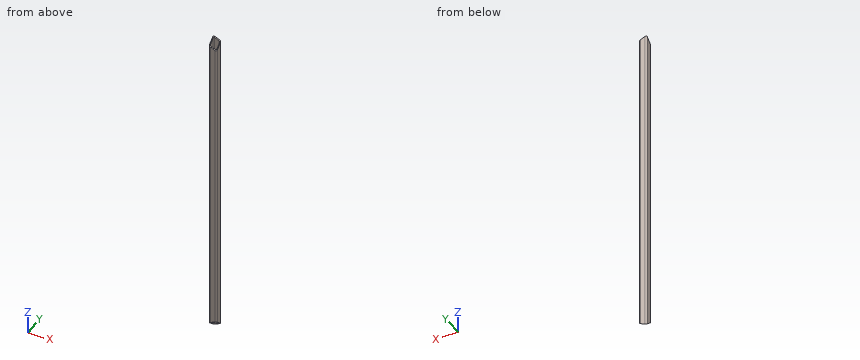
Autodesk Inventor part; units mm, degrees
ref_plane "Plano inicial" through (0, 0, -34.0777) normal (0, 0, 1) x (1, 0, 0)
ref_plane "Plano final" through (0, 0, 2032.731) normal (0, 0, 1) x (1, 0, 0)
ref_plane "Plano de trabalho4" through (-13.7846, 27.5692, -30.8233) normal (0.3162, -0.6325, -0.7071) x (0.6586, 0.6828, -0.3162)
ref_plane "Plano inicial" through (0, 0, -34.0777) normal (0, 0, 1) x (1, 0, 0)
ref_plane "Plano final" through (0, 0, 2032.731) normal (0, 0, 1) x (1, 0, 0)
sketch "Esboço" plane through (0, 0, 0) normal (0, 0, 1) x (1, 0, 0)
  line L0 (-25.4, -15.875) -> (-25.4, 15.875)
  line L1 (-15.875, 25.4) -> (15.875, 25.4)
  line L2 (25.4, 15.875) -> (25.4, -15.875)
  line L3 (15.875, -25.4) -> (-15.875, -25.4)
  arc A0 (-25.4, -15.875) -> (-15.875, -25.4) centre (-15.875, -15.875) ccw
  arc A1 (-15.875, 25.4) -> (-25.4, 15.875) centre (-15.875, 15.875) ccw
  arc A2 (25.4, 15.875) -> (15.875, 25.4) centre (15.875, 15.875) ccw
  arc A3 (15.875, -25.4) -> (25.4, -15.875) centre (15.875, -15.875) ccw
  arc A4 (-15.875, 20.6375) -> (-20.6375, 15.875) centre (-15.875, 15.875) ccw
  line L4 (-15.875, 20.6375) -> (15.875, 20.6375)
  arc A5 (20.6375, 15.875) -> (15.875, 20.6375) centre (15.875, 15.875) ccw
  line L5 (20.6375, 15.875) -> (20.6375, -15.875)
  arc A6 (15.875, -20.6375) -> (20.6375, -15.875) centre (15.875, -15.875) ccw
  line L6 (15.875, -20.6375) -> (-15.875, -20.6375)
  arc A7 (-20.6375, -15.875) -> (-15.875, -20.6375) centre (-15.875, -15.875) ccw
  line L7 (-20.6375, -15.875) -> (-20.6375, 15.875)
  line L8 (0, 38.3218) -> (0, -38.3218) construction
  line L9 (-38.3218, 0) -> (38.3218, 0) construction
  dimension "d10" = 50.8
  dimension "d11" = 50.8
  dimension "d12" = 4.7625
  dimension "d15" = 25.4
  dimension "d16" = 25.4
  dimension "d17" = 9.525
extrude "Corpo" add sketch "Esboço" along normal up to surface (2066.8087 mm away) from surface at -34.0777
sketch "Sketch3" plane through (0, 0, 0) normal (0, 0, 1) x (1, 0, 0)
  line L0 (0, 0) -> (10, 0)
ref_plane "Work Plane3" through (0, 0, 0) normal (0, -1, 0) x (1, 0, 0)
sketch "Sketch4" plane through (0, 0, 0) normal (0, -1, 0) x (1, 0, 0)
  line L0 (-2, -34.0777) -> (12, -34.0777)
  line L1 (-2, 2032.731) -> (12, 2032.731)
  dimension "d19" = 2066.8087
ref_plane "Plano de trabalho4" through (-13.7846, 27.5692, -30.8233) normal (0.3162, -0.6325, -0.7071) x (0.6586, 0.6828, -0.3162)
split "Dividir1" plane through (-13.7846, 27.5692, -30.8233) removes the side toward (0.3162, -0.6325, -0.7071)
ref_plane "Plano de trabalho5" through (-13.7846, 27.5692, 2029.6052) normal (0.3098, -0.6196, 0.7212) x (0.9442, 0.1115, -0.3098)
split "Dividir2" plane through (-13.7846, 27.5692, 2029.6052) removes the side toward (0.3098, -0.6196, 0.7212)
equation "\"d10\" = G_H"
equation "\"d11\" = G_W"
equation "\"d12\" = G_T"
equation "\"d15\" = 0.5 * d10"
equation "\"d16\" = 0.5 * d11"
equation "\"d17\" = G_IR"
equation "\"d3\" = G_L"
equation "\"G_W\" = 50.8"
equation "\"G_H\" = 50.8"
equation "\"G_T\" = 4.7625"
equation "\"G_IR\" = 9.525"
equation "\"G_L\" = 2060.38202"
equation "\"G_OFFSET_START\" = 34.07768"
equation "\"G_OFFSET_END\" = 32.73098"
equation "\"d13\" = -G_OFFSET_START"
equation "\"d14\" = G_OFFSET_END + B_L"
properties part number "AISC - 2 x 2 x 3/16 - 81,117" material "Aço, suave"
CAD build for the part. Positions are in the model's coordinates, mm. Coordinates: 2 decimals unless noted, no trailing zeros. Loops run counter-clockwise (first coordinate to the right, second up) from the corner with the lowest first, then second, coordinate; pieces in that order, holes last. Notation, with made-up numbers: (31.5, 33.25) -> (67.5, 33.25) arc R9 cw to (67.5, 47.25) -> close; hole circle Ø11 at (61.25, 74.5). An arc over 180 degrees is marked (long way). One line per item, written item: value.
1. Drill centre lines: line 1 (X direction, y = 16.5, z = 259); line 2 (Y direction, x = -14, z = 1445); line 3 (X direction, y = 22, z = 1805.5). Where is each one in solid material? Low to high. Write a range as [from, to].
Answers:
line 1: x = [-25.38, -20.6], [20.6, 25.38]
line 2: y = [-25.4, -20.64], [20.64, 25.4]
line 3: x = [-23.17, 23.17]
2. Flat gauge pins, fed straight in: P1, Ø4, axis at x = 13.5, y = -19.5, coming from the -Z side; P2, Ø2, axis at x = 3, y = -19.5, coming from the -Z side; P3, Ø2, axis at y = 18.5, z = 1084, coming from the +X side. Where does each tip first touch, or does it go through?
Answers:
P1: stops at z = 23.76
P2: passes through
P3: stops at x = 25.26
3. Slice it at A-A on x = 7. Write the cut outline in (y, z), and give its area (3 significant figures).
Answers:
outline: (-25.4, 25.85) -> (-20.64, 21.59) -> (-20.64, 1979.26) -> (-25.4, 1975.17) -> close; (20.64, -15.33) -> (25.4, -19.59) -> (25.4, 2018.81) -> (20.64, 2014.72) -> close
area: 19,000 mm^2
4. Slice it at C-C on y = -2. Write the cut outline in (x, z), and give its area (3 significant figures).
Answers:
outline: (-25.4, -9.57) -> (-20.64, -7.44) -> (-20.64, 2007.15) -> (-25.4, 2009.19) -> close; (20.64, 11.02) -> (25.4, 13.15) -> (25.4, 1987.37) -> (20.64, 1989.42) -> close
area: 19,000 mm^2
